Check sheet for the modelled part. Datum: model origin and axes. Units: mm. A direction names the side the tool comes from. Give positions to 0.01 mm unless a question says otherwise; leave off trailing zeros. Loops run counter-clockwise (first coordinate to the right, second up) from the corner with the lowest first, then second, coordinate; pieces in that order, holes last.
```python
from build123d import *

# Parameters (mm, degrees)
SKETCH1_R           = 4.5
BOSS_EXTRUDE1_DEPTH = 2.5
SKETCH2_R           = 2.45
BOSS_EXTRUDE2_DEPTH = 14
CHAMFER1_SIZE       = 2.5
CUT_EXTRUDE1_DEPTH  = 1.5


with BuildPart() as part:
    # Sketch1 → Boss-Extrude1 (new body)
    with BuildSketch(Plane(origin=(0, 0, 0), x_dir=(1, 0, 0), z_dir=(0, 1, 0))):
        with Locations(Location((0, 0, 0), (0, 0, 270))):
            Circle(SKETCH1_R)
    extrude(amount=BOSS_EXTRUDE1_DEPTH)

    # Sketch2 → Boss-Extrude2 (add)
    with BuildSketch(Plane(origin=(0, 2.5, 0), x_dir=(1, 0, 0), z_dir=(0, 1, 0))):
        with Locations(Location((0, 0, 0), (0, 0, 270))):
            Circle(SKETCH2_R)
    extrude(amount=BOSS_EXTRUDE2_DEPTH)

    # Chamfer1
    # the kernel refuses this chamfer: 2.5 mm, written as the material it takes off along each edge
    with BuildSketch(Plane(origin=(0, 2.5, 0), x_dir=(0, 0, 1), z_dir=(-1, 0, 0))) as chamfer1_piece_1_section:
        Polygon((4.5, -CHAMFER1_SIZE), (4.5 - CHAMFER1_SIZE, 0), (4.5, 0), align=None)
    chamfer1_piece_1 = revolve(axis=Axis((0, 2.5, 0), (0, 1, 0)), mode=Mode.PRIVATE)
    chamfer1_piece_1 = chamfer1_piece_1 - Plane(origin=(0, 1.019761833, 0), x_dir=(0, 0, 1), z_dir=(0, -1, 0)) * Cylinder(2.45, 18, mode=Mode.PRIVATE)
    add(chamfer1_piece_1, mode=Mode.SUBTRACT)

    # Sketch3 → Cut-Extrude1 (cut)
    with BuildSketch(Plane.XZ):
        Polygon((0, -1.662470902), (1.439742034, -0.831235451), (1.439742034, 0.831235451), (0, 1.662470902), (-1.439742034, 0.831235451), (-1.439742034, -0.831235451), align=None)
    extrude(amount=-CUT_EXTRUDE1_DEPTH, mode=Mode.SUBTRACT)


solid = part.part
```
(1) Section check B-B on y = 6. Record the boundary of the cut face in (x, z).
(2) Access from +Z, -Z, +X, -X, +Y, -Y to the whole of each face (thin tool, end or side, straight path). Record for faces 4 (the face through (-2, 0, 0)), 5 (the face through (-0.71, 0.74, 1.253)).
(3) Gauge pin test, flat ends, axial feed: pin 1 Ø1.2 at (y, z) = (1, 0) entering from +X; pin 2 Ø1 at (x, y) = (-0.5, 13.5) entering from -Z; pin 3 Ø5 at (x, z) = (0.5, -3) entering from +Y; pin 4 Ø1.5 at (y, z) = (11, 2.5) entering from -X. Record the tip position at first contact, or that the pin passes through.
(4) Release check for a two-part mould opening along Z. For faces 1 (the face through (2.4, 9.2, -0.5)), 2 (the face through (-0.73, 0.74, -1.24)), 3 (the face through (0, 16.5, 0)) record: pulls with the +Z half, pulls with the -Z half, needs draft (parallel to the pull), parting line crosses it, or undercut.
(5) Material ranges on line 1 (Y direction, x = -2.75, z = 0.5); line 2 (X direction, y = 14.25, z = -2); line 3 (X direction, y = 14, z = 1.75), recorded low to high.
(6) Section check A-A on z = 0. Record the boundary of the cut face in (x, y), plus the area to 3 significant figures.
Computed values:
1. outline: circle Ø4.9 at (0, 0)
2. face 4: +Z, -Z, +X, -X, -Y
2. face 5: -Y
3. pin 1: stops at x = 4.1
3. pin 2: stops at z = -2.45
3. pin 3: stops at y = 16.5
3. pin 4: stops at x = -1.71
4. face 1: parting line crosses it
4. face 2: undercut
4. face 3: needs draft
5. line 1: y = 0 to 1.7
5. line 2: x = -1.42 to 1.42
5. line 3: x = -1.71 to 1.71
6. outline: (-4.5, 0) - (-1.44, 0) - (-1.44, 1.5) - (1.44, 1.5) - (1.44, 0) - (4.5, 0) - (2.45, 2.05) - (2.45, 16.5) - (-2.45, 16.5) - (-2.45, 2.05) - close
6. area: 80.7 mm2
